Design review of the part shown in the three views and the two pictorial views. Dimensions are in mm from the part's minimum x, y and z. A direction names the side the tool comes from. Round coordinates to 2 decimals unless told otherwise and drop trailing zeros. Write each loop counter-clockwise with the first axis right and the second up, starting at its lowest first coordinate (ties: lowest second). Pieces come first, ordered by that corner, then holes. Notation, with made-up numbers: (26.25, 15) -> (49.25, 15) arc R27 cw to (49.25, 50) -> close; hole circle Ø4 at (78, -29.5). An arc over 180 degrees is marked (long way). Return JSON: item names as keys, results as strings. Group by question number.
1. Take a section at D-D, the plane y = 45. Write out the cut boundary in (x, z).
2. Mouldability with a two-part tool opening along X and no side actions: class the marked faces 1, 2 and 3 as pulls with the +X half, pulls with the -X half, needs draft (parallel to the pull), parting line crosses it, or undercut.
3. Take a section at C-C, the plane z = 11.25. Write out the cut boundary in (x, y), then the cut area to 3 significant figures.
4. Take a section at A-A, the plane x = 43.15. Write out the cut boundary in (y, z), then the cut area to 3 significant figures.
5. Clearance check with flat-ended pins moving along their axes: P1, Ø4, axis at x = 10, y = 47, coming from the +Z side; P2, Ø12, axis at x = 6, y = 7, coming from the -Z side. State where each tip first meets the part, or that it passes through.
6. Take a section at B-B, the plane y = 9.5. Write out the cut boundary in (x, z).
7. Tool access review of the marked faces 4 and 5: name each direction out of +Z, -Z, +X, -X, +Y, -Y from which nothing blocks a thin tool from reaching the whole face with its end or side.
8. For line 1 along Z through (x, y) = (43.15, 1.1); line 2 along X through (y, z) = (42.5, 27.5); line 3 along Y through (x, z) = (50.5, 10), list the stretches that pass through material, from the lowest coordinate up. Write a range as from..to.
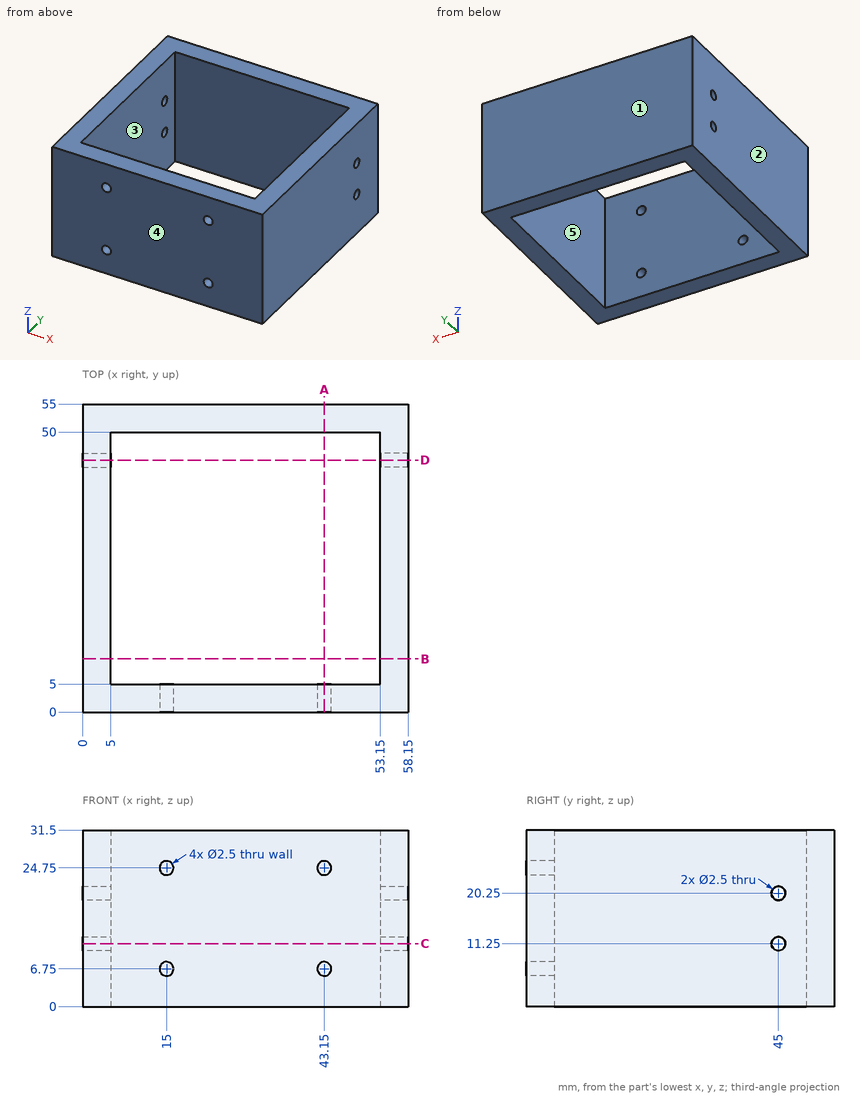
Output:
{
 "1": {"outline": "(0, 0) -> (5, 0) -> (5, 10) -> (0, 10) -> close; (0, 12.5) -> (5, 12.5) -> (5, 19) -> (0, 19) -> close; (0, 21.5) -> (5, 21.5) -> (5, 31.5) -> (0, 31.5) -> close; (53.15, 0) -> (58.15, 0) -> (58.15, 10) -> (53.15, 10) -> close; (53.15, 12.5) -> (58.15, 12.5) -> (58.15, 19) -> (53.15, 19) -> close; (53.15, 21.5) -> (58.15, 21.5) -> (58.15, 31.5) -> (53.15, 31.5) -> close"},
 "2": {"face 1": "needs draft", "face 2": "pulls with the -X half", "face 3": "undercut"},
 "3": {"outline": "(0, 0) -> (58.15, 0) -> (58.15, 43.75) -> (53.15, 43.75) -> (53.15, 5) -> (5, 5) -> (5, 43.75) -> (0, 43.75) -> close; (0, 46.25) -> (5, 46.25) -> (5, 50) -> (53.15, 50) -> (53.15, 46.25) -> (58.15, 46.25) -> (58.15, 55) -> (0, 55) -> close", "area": "1,010 mm^2"},
 "4": {"outline": "(0, 0) -> (5, 0) -> (5, 5.5) -> (0, 5.5) -> close; (0, 8) -> (5, 8) -> (5, 23.5) -> (0, 23.5) -> close; (0, 26) -> (5, 26) -> (5, 31.5) -> (0, 31.5) -> close; (50, 0) -> (55, 0) -> (55, 31.5) -> (50, 31.5) -> close", "area": "290 mm^2"},
 "5": {"P1": "passes through", "P2": "stops at z = 0"},
 "6": {"outline": "(0, 0) -> (5, 0) -> (5, 31.5) -> (0, 31.5) -> close; (53.15, 0) -> (58.15, 0) -> (58.15, 31.5) -> (53.15, 31.5) -> close"},
 "7": {"face 4": "+Z, -Z, +X, -X, -Y", "face 5": "+Z, -Z"},
 "8": {"line 1": "z = 0..5.5, 8..23.5, 26..31.5", "line 2": "x = 0..5, 53.15..58.15", "line 3": "y = 0..5, 50..55"}
}
